Geometry check sheet. Reference: the model listing, model coordinates, mm. Face numbers are marked on the shaded views. A direction names the side the tool comes from. Give positions to 0.01 mm unless a question says otherwise; leave off trailing zeros. Loops run counter-clockwise (first coordinate to the right, second up) from the corner with the lowest first, then second, coordinate; pieces in that order, holes last. Notation, with made-up numbers: (72, -21.75) -> (84, -21.75) arc R17 cw to (84, 7.25) -> close; hole circle Ø5 at (47, 26.5). An arc over 180 degrees is marked (long way). Answer as a JSON object with one key per item and string values.
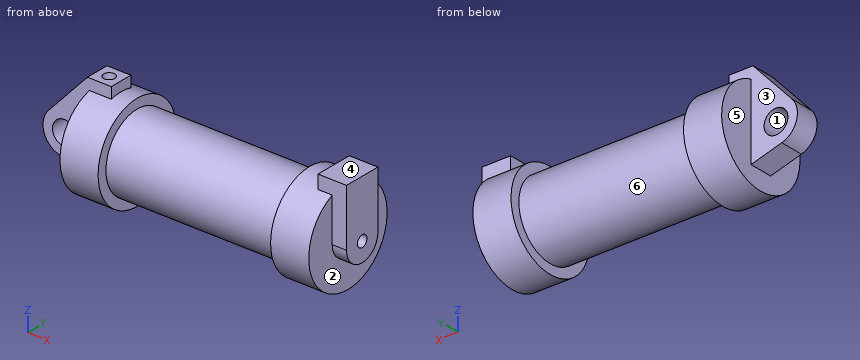
from build123d import *

# Parameters (mm, degrees)
F0_R     = 3.175
F0_W     = 5.842
F0_H     = 12.7
F2_DEPTH = 3.175
F4_R     = 1.524
F5_DEPTH = 3.81
F7_R     = 1.524
F9_DEPTH = 17.78


# Not quite as in the source:
# - the program builds the solid bodies; features that only make, move or delete a surface that nothing else refers to are left out


with BuildPart() as f1:
    # F0 (on Front) → F1 (revolve)
    with BuildSketch(Plane.XZ):
        Polygon((5.842, 12.7), (5.842, 0), (66.294, 0), (66.294, 12.7), (56.134, 12.7), (56.134, 10.16), (10.16, 10.16), (10.16, 12.7), align=None)
    revolve(axis=Axis((33.147, 0, 0), (-1, 0, 0)))

    # F0 (on Front) → F2 (join, symmetric)
    with BuildSketch(Plane.XZ):
        with BuildLine():
            Line((5.842, 0), (0, 0))
            Line((0, 0), (-0.9398, 0))
            ThreePointArc((-0.9398, 0), (-3.1957909266, -4.5493385486), (-8.1826630726, -5.5069827884))
            Line((-8.1826630726, -5.5069827884), (5.842, -9.398))
            Line((5.842, -9.398), (5.842, 0))
        make_face()
        with BuildLine():
            ThreePointArc((-8.1826630726, -5.5069827884), (-3.1957909266, -4.5493385486), (-0.9398, 0))
            ThreePointArc((-0.9398, 0), (-4.5919612295, 5.3297205562), (-10.8806298187, 3.8475430269))
            ThreePointArc((-10.8806298187, 3.8475430269), (-12.1459778134, -1.5837270034), (-8.1826630726, -5.5069827884))
        make_face()
        with Locations((-6.6548, 0)):
            Circle(F0_R, mode=Mode.SUBTRACT)
        with BuildLine():
            Line((-0.9398, 0), (0, 0))
            Line((0, 0), (0, 12.7))
            Line((0, 12.7), (5.842, 12.7))
            Line((5.842, 12.7), (5.842, 15.24))
            Line((5.842, 15.24), (-0.508, 15.24))
            Line((-0.508, 15.24), (-10.8806298187, 3.8475430269))
            ThreePointArc((-10.8806298187, 3.8475430269), (-4.5919612295, 5.3297205562), (-0.9398, 0))
        make_face()
        with Locations((2.921, 6.35)):
            Rectangle(F0_W, F0_H)
    extrude(amount=F2_DEPTH, both=True)

    # F0 (on Front) → F3 (revolve)
    with BuildSketch(Plane.XZ):
        with Locations((2.921, 6.35)):
            Rectangle(F0_W, F0_H)
    revolve(axis=Axis((33.147, 0, 0), (-1, 0, 0)))

    # F4 (on face) → F5 (join, symmetric)
    with BuildSketch(Plane.YZ.offset(66.294)):
        with BuildLine():
            ThreePointArc((-5.08, 0), (0, -5.08), (5.08, 0))
            ThreePointArc((5.08, 0), (0, 5.08), (-5.08, 0))
        make_face()
        Circle(F4_R, mode=Mode.SUBTRACT)
        with BuildLine():
            ThreePointArc((-5.08, 0), (0, 5.08), (5.08, 0))
            Line((5.08, 0), (5.08, 11.6397422652))
            ThreePointArc((5.08, 11.6397422652), (0, 12.7), (-5.08, 11.6397422652))
            Line((-5.08, 11.6397422652), (-5.08, 0))
        make_face()
        with BuildLine():
            ThreePointArc((-5.08, 11.6397422652), (0, 12.7), (5.08, 11.6397422652))
            Line((5.08, 11.6397422652), (5.08, 15.24))
            Line((5.08, 15.24), (-5.08, 15.24))
            Line((-5.08, 15.24), (-5.08, 11.6397422652))
        make_face()
    extrude(amount=F5_DEPTH, both=True)

    # F7 (on face) → F9 (cut)
    with BuildSketch(Plane.XY.offset(15.24)):
        with Locations((2.667, 0)):
            Circle(F7_R)
    extrude(amount=-F9_DEPTH, mode=Mode.SUBTRACT)


solid = f1.part
1) Section check D-D on x = 2. Record the cut outline in (y, z) (3 decimals), plus the area to 3 significant figures.
Geometry check:
{"outline": "(-3.175, 12.297) arc R12.7 ccw (long way) to (3.175, 12.297) -> (3.175, 15.24) -> (1.37, 15.24) -> (1.37, -2.54) -> (-1.37, -2.54) -> (-1.37, 15.24) -> (-3.175, 15.24) -> close", "area": "475 mm2"}
2) Section check C-C on x = 33.5. Record the cut outline in (y, z), plus the area to 3 significant figures.
Geometry check:
{"outline": "circle Ø20.32 at (0, 0)", "area": "324 mm2"}
3) Material ranges on line 1 along Y through (x, z) = (67.15, 0); line 2 along Z through (x, y) = (69.15, 0); line 3 along X through (y, z) = (-9, 7.75), recorded low to high. Write a range as from..to.
Geometry check:
{"line 1": "y = -5.08..-1.52, 1.52..5.08", "line 2": "z = -5.08..-1.52, 1.52..15.24", "line 3": "x = 0..10.16, 56.13..66.29"}
4) Depth check by flat-ended pin: P1, Ø9, axis at x = 1.5, z = 9, coming from the +Y side; P2, Ø3, axis at x = 8, z = -5, coming from the +Y side; P3, Ø1.5, axis at y = 0, z = 0, coming from the +X side. Enter the tip coordinate at first touch or a pass-through.
Geometry check:
{"P1": "stops at y = 11.88", "P2": "stops at y = 12.21", "P3": "stops at x = 66.29"}
5) Draft check along X on the marked faces 1, 2 and 3. Enter one of: pulls with the +X half, pulls with the -X half, needs draft (parallel to the pull), parting line crosses it, or undercut.
Geometry check:
{"face 1": "undercut", "face 2": "pulls with the +X half", "face 3": "needs draft"}
6) Tool access check on the marked faces 4, 5 and 6. Record the directions out of +Z, -Z, +X, -X, +Y, -Y that give a thin tool (end or side, any length) a straight path to the whole face; none if there is none.
Geometry check:
{"face 4": "+Z, +X, -X, +Y, -Y", "face 5": "-Z, -X", "face 6": "none"}
7) Section check B-B on y = 7.5. Record the cut outline in (x, z).
Geometry check:
{"outline": "(0, -10.25) -> (10.16, -10.25) -> (10.16, -6.85) -> (56.13, -6.85) -> (56.13, -10.25) -> (66.29, -10.25) -> (66.29, 10.25) -> (56.13, 10.25) -> (56.13, 6.85) -> (10.16, 6.85) -> (10.16, 10.25) -> (0, 10.25) -> close"}
